Here's how the part is built. I have some questions about the finished solid (model axes, mm). Face numbers are marked on the shaded views. Give positions to 0.01 mm unless a question says otherwise; leave off trailing zeros. Loops run counter-clockwise (first coordinate to the right, second up) from the corner with the lowest first, then second, coordinate; pieces in that order, holes last. Notation, with made-up numbers: M 6,18.5 L 18,18.5 A14 cw 18,24.5 Z; hole C 11.25,45 d9. An arc over 180 degrees is marked long. Write item = value, one per line. Start each with the question number.
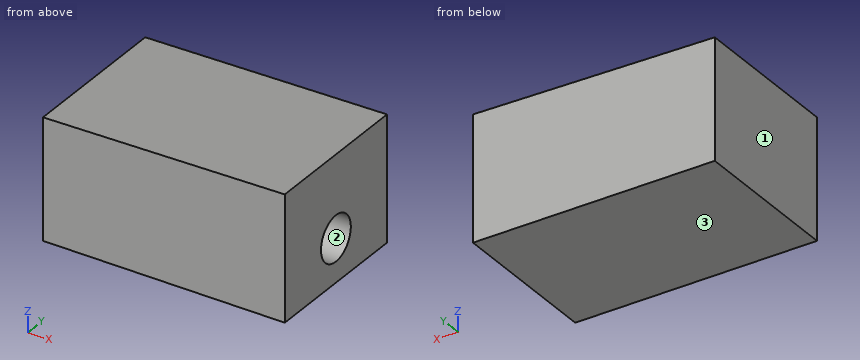
```python
from build123d import *

# Parameters (mm, degrees)
F1_DEPTH = 57.15
F3_D     = 16.66748
F3_DEPTH = 58.42
F3_TIP   = 5.0074161752


with BuildPart() as f1:
    # F0 (on Front) → F1 (new body)
    with BuildSketch(Plane.XZ):
        Polygon((0, 44.2722), (0, 0), (88.9, 0), (88.9, 45.974), align=None)
    extrude(amount=F1_DEPTH)

    # F3
    with Locations(Plane.YZ.offset(88.9)):
        with Locations((-28.575, 15.875)):
            Hole(F3_D / 2, depth=F3_DEPTH)
            with Locations((0, 0, -(F3_DEPTH + F3_TIP / 2))):  # 118° drill point
                Cone(0, F3_D / 2, F3_TIP, mode=Mode.SUBTRACT)


solid = f1.part
```
Q1. If I drill on line 1 along Y through (x, z) = (78, 19.5); line 2 along Z through (x, y) = (50.5, -26.5); line 3 along Z through (x, y) = (68.5, -34), over which ranges is the centre line in solid material (lowest first)?
Q2. We'd pull the mould along Z, two halves only. Please class the marked faces 1, 2 and 3: pulls with the +Z half, pulls with the -Z half, needs draft (parallel to the pull), parting line crosses it, or undercut.
Q3. Will these pins go through, and if not, where does the flat tip stop? pin 1 (8 mm diameter, centred on x = 62.5, y = -19.5, fed in from -Z); pin 2 (12 mm diameter, centred on x = 57, y = -43.5, fed in from +Z); pin 3 (10 mm diameter, centred on y = -28.575, z = 15.875, fed in from +X).
Q4. If we section it at B-B, the plane x = 83.5: List the corners of the cut face in (y, z) for me (3 decimals).
Q5. If we section it at A-A, the plane y = -46: List the corners of the cut face in (x, z) for me.
Q6. If we section it at C-C, the plane x = 19: List the corners of the cut face in (y, z) for me, then the cut area to 3 significant figures.
Q7. If we section it at D-D, the plane x = 58: List the corners of the cut face in (y, z) for me (3 decimals), then the cut area to 3 significant figures.
Resolved:
q1.line_1 = -57.15 to -36.08, -21.07 to 0
q1.line_2 = 0 to 7.8, 23.95 to 45.24
q1.line_3 = 0 to 9.55, 22.2 to 45.58
q2.face_1 = needs draft
q2.face_2 = undercut
q2.face_3 = pulls with the -Z half
q3.pin_1 = 0
q3.pin_2 = 45.48
q3.pin_3 = 28.48
q4.outline = M -57.15,0 L 0,0 L 0,45.871 L -57.15,45.871 Z; hole C -28.575,15.875 d16.667
q5.outline = M 0,0 L 88.9,0 L 88.9,45.97 L 0,44.27 Z
q6.outline = M -57.15,0 L 0,0 L 0,44.64 L -57.15,44.64 Z
q6.area = 2,550 mm²
q7.outline = M -57.15,0 L 0,0 L 0,45.382 L -57.15,45.382 Z; hole C -28.575,15.875 d16.667
q7.area = 2,380 mm²
